```python
from build123d import *

# Parameters (mm, degrees)
SKETCH1_R           = 38.1
SKETCH1_R_2         = 9.525
BOSS_EXTRUDE1_DEPTH = 12.7
SKETCH2_R           = 4.445
CUT_EXTRUDE1_DEPTH  = 56.358016583
CIRPATTERN1_COUNT   = 21


with BuildPart() as part:
    # Sketch1 → Boss-Extrude1 (new body)
    with BuildSketch(Plane.XY):
        Circle(SKETCH1_R)
        Circle(SKETCH1_R_2, mode=Mode.SUBTRACT)
    extrude(amount=BOSS_EXTRUDE1_DEPTH)

    # Sketch2 → Cut-Extrude1 (cut, through all)
    with BuildSketch(Plane.XY.offset(12.7)):
        with Locations((0, 38.1)):
            Circle(SKETCH2_R)
    cut_extrude1 = extrude(amount=-CUT_EXTRUDE1_DEPTH, mode=Mode.SUBTRACT)

    # CirPattern1: Cut-Extrude1 ×21 about axis
    cirpattern1_axis = Axis((0, 0, 0), (0, 0, 1))
    for i in range(1, CIRPATTERN1_COUNT):
        add(cut_extrude1.rotate(cirpattern1_axis, i * 360 / CIRPATTERN1_COUNT), mode=Mode.SUBTRACT)


solid = part.part
```
Source: CAD feature listing. Evaluate the final solid. Frame: model axes, mm. Coordinates: 2 decimals unless noted, no trailing zeros. Loops run counter-clockwise (first coordinate to the right, second up) from the corner with the lowest first, then second, coordinate; pieces in that order, holes last. Notation, with made-up numbers: M 4.5,-10 L 50.5,-10 A17 ccw 50.5,0 Z; hole C -14,47.5 d1. An arc over 180 degrees is marked long. Put each result on its own line as item: value. Start each with the question number.
1) Cut plane C-C on y = -19.05. Return the cut outline in (x, z), then the cut area to 3 significant figures.
2) Contact query for flat-ended pins moving along their axis: pin 1 Ø5 at (y, z) = (-15.5, 7.5) entering from +X; pin 2 Ø1 at (x, z) = (13.5, 11) entering from +Y; pin 3 Ø3 at (x, y) = (-8, 23.5) entering from -Z; pin 4 Ø1.5 at (x, z) = (18, 7) entering from +Y. Output: stop coordinate, or through.
3) Cut plane D-D on x = 11. Return the cut outline in (y, z), then the cut area to 3 significant figures.
4) Cut plane B-B on y = 0. Return the cut outline in (x, z) (3 decimals), then the cut area to 3 significant figures.
5) Ray query, L1, parallel to Y at x = 0, z = 8 (3 decimals); L2, parallel to Y at x = -33.5, z = 9.25; L3, parallel to X at y = 20, z = 6. Return the intervals inside material, ascending. Write a range as from..to.
6) Pull-direction query (Y, two-part tool) for faces 1 (the face through (37.992, -2.865, 6.261)), 2 (the face through (-32.79, -7.58, 6.44)), 3 (the face through (-25.902, 27.941, 6.261)); classes: pulls with the +Y half, pulls with the -Y half, needs draft (parallel to the pull), parting line crosses it, or undercut.
7) Cut plane A-A on x = 0. Return the cut outline in (y, z) (3 decimals).
The answers:
1. outline: M -28.55,0 L 28.55,0 L 28.55,12.7 L -28.55,12.7 Z
1. area: 725 mm²
2. pin 1: stops at x = 35.81
2. pin 2: stops at y = 32.93
2. pin 3: stops at z = 0
2. pin 4: stops at y = 33.97
3. outline: M -36.48,0 L 31.97,0 L 31.97,12.7 L -36.48,12.7 Z
3. area: 869 mm²
4. outline: M -34.58,0 L -9.525,0 L -9.525,12.7 L -34.58,12.7 Z; M 9.525,0 L 34.58,0 L 34.58,12.7 L 9.525,12.7 Z
4. area: 636 mm²
5. L1: y = -38.1..-9.525, 9.525..33.655
5. L2: y = -14.63..-11.02, -5.93..9.93, 17.91..18.15
5. L3: x = -32.43..-32.17, -27.41..27.41, 32.17..32.43
6. face 1: pulls with the -Y half
6. face 2: undercut
6. face 3: pulls with the +Y half
7. outline: M -38.1,0 L -9.525,0 L -9.525,12.7 L -38.1,12.7 Z; M 9.525,0 L 33.655,0 L 33.655,12.7 L 9.525,12.7 Z
